Can you work these out from the model? Positions are in its coordinate system, mm. Coordinates: 2 decimals unless noted, no trailing zeros. Order: outer loops, then holes, each group sorted by start corner. A loop starts at its lowest first (then second) coordinate and runs counter-clockwise, first axis right, second up. Notation, with made-up numbers: (80, 21) -> (91, 21) arc R13 ccw to (91, 39) -> close; hole circle Ø9 at (34.5, 3.25). An arc over 180 degrees is marked (long way). Return JSON: item names as keys, results as strings. Group by question number.
1) If I drill on probe 1 along Y at (x, z) = (20, 2.1); probe 2 along X at (y, z) = (-153, 4.15); probe 3 along Y at (x, z) = (-8, 2.55), over which ranges is the centre line in solid material (lowest first)? Write a range as from..to.
2) If we section it at C-C, the plane y = -153: Please give me the cut outline in (x, z).
3) For pin 1 (2 mm diameter, centred on y = -115.5, z = 0.5, fed in from +X); pin 2 (2 mm diameter, centred on x = 101, z = 0.5, fed in from -Y); pin 3 (2 mm diameter, centred on y = -144.5, z = 1.5, fed in from +X); pin 4 (10 mm diameter, centred on x = 34.5, y = 37, fed in from -Z), each with a flat end and sliding along its axis, tell me the tip position at first contact or that it passes through.
4) If we section it at A-A, the plane z = 2.1: Please give me the cut outline in (x, y) (3 decimals).
5) If we section it at B-B, the plane x = 105: Please give me the cut outline in (y, z), then the cut area to 3 significant figures.
from build123d import *

# Parameters (mm, degrees)
SKETCH1_W           = 254
SKETCH1_H           = 457.2
BOSS_EXTRUDE1_DEPTH = 4.3434
CUT_EXTRUDE3_DEPTH  = 5.3434
FILLET2_R           = 1.27


with BuildPart() as part:
    # Sketch1 → Boss-Extrude1 (new body)
    with BuildSketch(Plane.XY):
        Rectangle(SKETCH1_W, SKETCH1_H)
    extrude(amount=BOSS_EXTRUDE1_DEPTH)

    # Sketch4 → Cut-Extrude3 (cut, through all)
    with BuildSketch(Plane.XY.offset(4.3434)):
        Polygon((-127, -228.6), (127, -81.953031626), (127, -228.6), align=None)
    extrude(amount=-CUT_EXTRUDE3_DEPTH, mode=Mode.SUBTRACT)

    # Fillet2
    fillet2_edges = [part.edges().sort_by_distance(p)[0] for p in [
        (127, -81.953031626, 2.1717),
        (-127, -228.6, 2.1717),
        (-127, 228.6, 2.1717),
        (127, 228.6, 2.1717),
    ]]
    fillet(fillet2_edges, radius=FILLET2_R)


solid = part.part
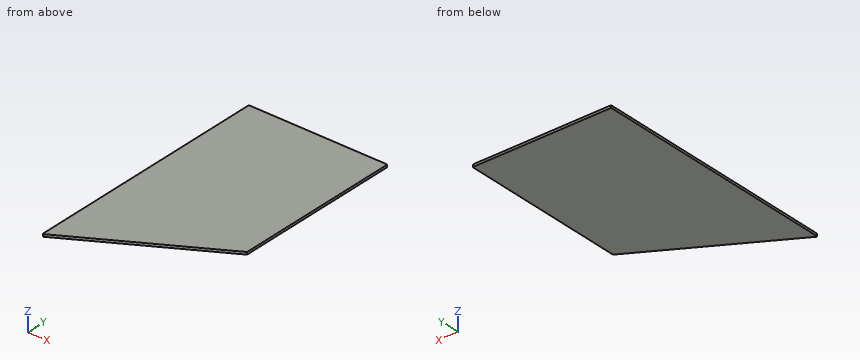
Result sheet:
{
 "1": {"probe 1": "y = -143.73..228.6", "probe 2": "x = -127..3.94", "probe 3": "y = -159.9..228.6"},
 "2": {"outline": "(-127, 0) -> (3.94, 0) -> (3.94, 4.34) -> (-127, 4.34) -> close"},
 "3": {"pin 1": "stops at x = 70.63", "pin 2": "stops at y = -97.54", "pin 3": "stops at x = 20.4", "pin 4": "stops at z = 0"},
 "4": {"outline": "(-127, -226.4) arc R1.27 ccw to (-125.095, -227.5) -> (126.365, -82.32) arc R1.27 ccw to (127, -81.22) -> (127, 227.33) arc R1.27 ccw to (125.73, 228.6) -> (-125.73, 228.6) arc R1.27 ccw to (-127, 227.33) -> close"},
 "5": {"outline": "(-94.65, 0) -> (228.6, 0) -> (228.6, 4.34) -> (-94.65, 4.34) -> close", "area": "1,400 mm2"}
}
